from build123d import *

# Parameters (mm, degrees)
F0_W     = 22.098
F0_H     = 47.498
F1_DEPTH = 685.8
F2_R     = 3.9751
F3_DEPTH = 1.651
F4_R     = 9.525
F5_DEPTH = 1.651


with BuildPart() as f1:
    # F0 (on Front) → F1 (new body)
    with BuildSketch(Plane.XZ):
        with BuildLine():
            ThreePointArc((0, 1.651), (0.483567, 0.483567), (1.651, 0))
            Line((1.651, 0), (23.749, 0))
            ThreePointArc((23.749, 0), (24.916433, 0.483567), (25.4, 1.651))
            Line((25.4, 1.651), (25.4, 49.149))
            ThreePointArc((25.4, 49.149), (24.916433, 50.316433), (23.749, 50.8))
            Line((23.749, 50.8), (1.651, 50.8))
            ThreePointArc((1.651, 50.8), (0.483567, 50.316433), (0, 49.149))
            Line((0, 49.149), (0, 1.651))
        make_face()
        with Locations((12.7, 25.4)):
            Rectangle(F0_W, F0_H, mode=Mode.SUBTRACT)
    extrude(amount=F1_DEPTH)

    # F2 (on face) → F3 (cut, through all)
    with BuildSketch(Plane.YZ.offset(25.4)):
        with Locations((-50.8, 25.4)):
            Circle(F2_R)
    extrude(amount=-F3_DEPTH, mode=Mode.SUBTRACT)

    # F4 (on face) → F5 (cut, through all)
    with BuildSketch(Plane(origin=(0, 0, 0), x_dir=(0, -1, 0), z_dir=(-1, 0, 0))):
        with Locations((50.8, 25.4)):
            Circle(F4_R)
    extrude(amount=-F5_DEPTH, mode=Mode.SUBTRACT)


solid = f1.part
Part model, mm, in its own coordinate system. A direction names the side the tool comes from. Give positions to 0.01 mm unless a question says otherwise; leave off trailing zeros. Order: outer loops, then holes, each group sorted by start corner. A loop starts at its lowest first (then second) coordinate and runs counter-clockwise, first axis right, second up. Notation, with made-up numbers: (-13, 45.25) - (10, 45.25) arc R22 cw to (10, 83.25) - close; hole circle Ø6 at (22, 6). An arc over 180 degrees is marked (long way). One line per question, with ' | ' between items.
1. Pull direction X, two halves, no side cores. Call faces 4 (the face through (25.4, -338, 25)), 5 (the face through (13, -338, 1.651)), 6 (the face through (13, -338, 50.8)), 7 (the face through (0, -338, 26)): +X half, -X half, draft (parallel to the pull), parting line (faces both ways), or undercut.
Filled in:
face 4: +X half | face 5: undercut | face 6: draft | face 7: -X half
2. Band-saw the part on C-C on x = 10.75. List the corners of the cut face in (y, z).
Filled in:
outline: (-685.8, 0) - (0, 0) - (0, 1.65) - (-685.8, 1.65) - close; (-685.8, 49.15) - (0, 49.15) - (0, 50.8) - (-685.8, 50.8) - close
3. Band-saw the part on A-A on y = -380. List the corners of the cut face in (x, z), then the cut area to 3 significant figures.
Filled in:
outline: (0, 1.65) arc R1.65 ccw to (1.65, 0) - (23.75, 0) arc R1.65 ccw to (25.4, 1.65) - (25.4, 49.15) arc R1.65 ccw to (23.75, 50.8) - (1.65, 50.8) arc R1.65 ccw to (0, 49.15) - close; hole (1.65, 1.65) - (23.75, 1.65) - (23.75, 49.15) - (1.65, 49.15) - close | area: 238 mm²
4. Band-saw the part on B-B on z = 41.5. List the corners of the cut face in (x, y).
Filled in:
outline: (0, -685.8) - (1.65, -685.8) - (1.65, 0) - (0, 0) - close; (23.75, -685.8) - (25.4, -685.8) - (25.4, 0) - (23.75, 0) - close
5. Drill centre lines: probe 1 along Z at (x, y) = (24.3, -50.8); probe 2 along X at (y, z) = (-125.5, 5.5); probe 3 along Z at (x, y) = (6.75, -640.5). Where is each one in solid material? Low to high.
Filled in:
probe 1: 0.09 to 21.42, 29.38 to 50.71 | probe 2: 0 to 1.65, 23.75 to 25.4 | probe 3: 0 to 1.65, 49.15 to 50.8
6. Which spindle directions (+Z, -Z, +X, -X, +Y, -Y) get a long thin tool onto all of the face, cutting with end or side? Do faces 1 (the face through (23.749, -338, 25)), 2 (the face through (0.81, -55.2, 16.95)), 3 (the face through (1, -685.8, 27)). Say none if no direction does.
Filled in:
face 1: +Y, -Y | face 2: -X | face 3: +Z, -Z, +X, -X, -Y
